Print and shaded views of the part. All mm, measured from the part's lowest x, y and z. A direction names the side the tool comes from. Round coordinates to 2 decimals unless told otherwise and drop trailing zeros. Order: outer loops, then holes, each group sorted by start corner. A loop starts at its lowest first (then second) coordinate and runs counter-clockwise, first axis right, second up. Notation, with made-up numbers: (77.25, 78.5) - (119.25, 78.5) arc R7 cw to (119.25, 82.5) - close; hole circle Ø5 at (51.25, 75). An arc over 180 degrees is marked (long way). Return JSON: item names as keys, results as strings. Group by question number.
Item 1: Saw through at C-C on z = 5. List the corners of the cut face in (x, y).
Item 2: Tool access for the marked faces 1, 2, 3, 4 and 5: list every direction of +Z, -Z, +X, -X, +Y, -Y with a clear straight run to the whole face (end or side of a thin tool).
Item 3: Saw through at A-A on x = 41. State how many separate pieces and enclosed holes the cut face has, and give its area (3 significant figures).
Item 4: Drop flat-ended pins along their axis: pin 1 (4 mm diameter, centred on x = 26.5, y = 19, fed in from +Z); pin 2 (3 mm diameter, centred on x = 8.5, y = 4, fed in from -Z); pin 3 (8 mm diameter, centred on x = 6.5, z = 33.5, fed in from -Y). Give the stop position or say it passes through.
Item 5: Saw through at B-B on y = 9. List the corners of the cut face in (x, z).
Item 6: Saw through at D-D on z = 30. List the corners of the cut face in (x, y).
Item 7: Probe probe 1 along Z at (x, y) = (21, 13.25); probe 2 along Y at (x, z) = (26.5, 19.5). List the from-to ranges inside material, lowest first.
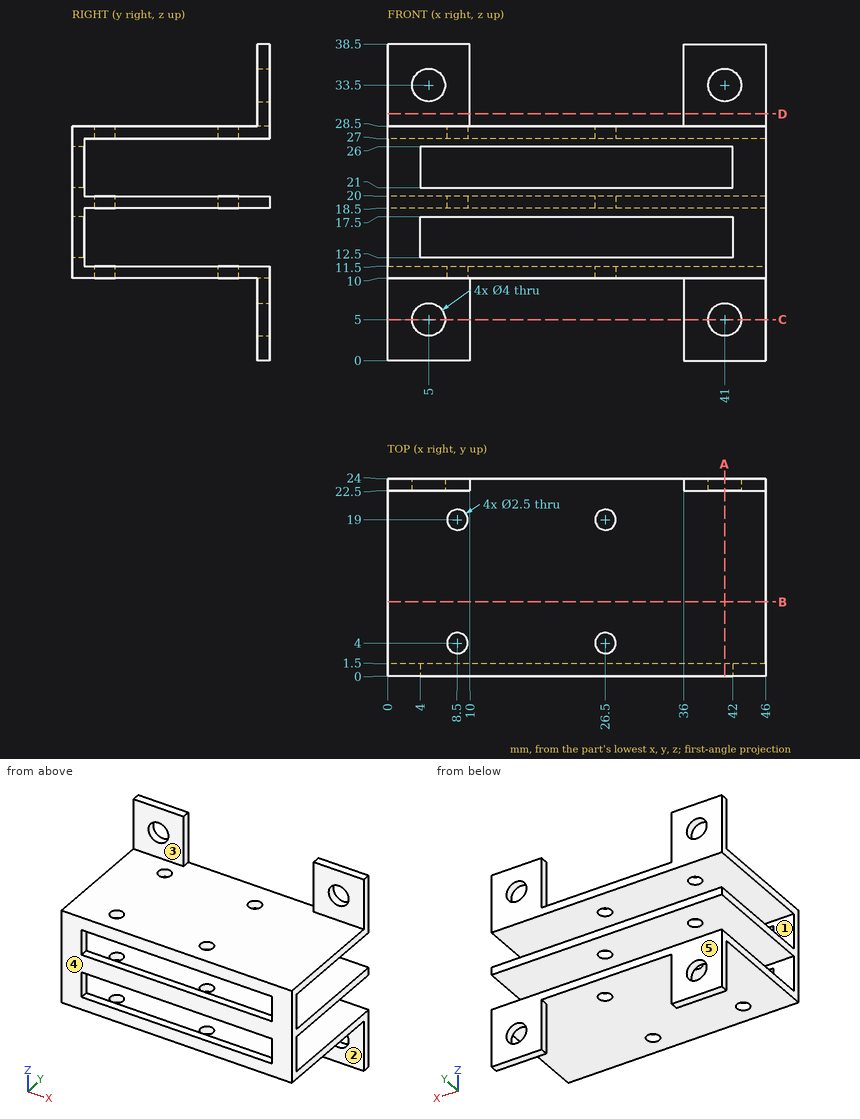
Filled in:
{
 "1": {"outline": "(0, 22.5) - (3, 22.5) - (3, 24) - (0, 24) - close; (7, 22.5) - (10, 22.5) - (10, 24) - (7, 24) - close; (36, 22.5) - (39, 22.5) - (39, 24) - (36, 24) - close; (43, 22.5) - (46, 22.5) - (46, 24) - (43, 24) - close"},
 "2": {"face 1": "+X, -X, +Y", "face 2": "-Z, +X, -X, -Y", "face 3": "+Z, +X, -X, -Y", "face 4": "+Z, -Z, +X, -X, -Y", "face 5": "+Z, -Z, +X, -X, +Y"},
 "3": {"separate pieces": "5", "enclosed holes": "0", "area": "132 mm^2"},
 "4": {"pin 1": "stops at z = 28.5", "pin 2": "stops at z = 10", "pin 3": "stops at y = 22.5"},
 "5": {"outline": "(0, 10) - (46, 10) - (46, 11.5) - (0, 11.5) - close; (0, 18.5) - (46, 18.5) - (46, 20) - (0, 20) - close; (0, 27) - (46, 27) - (46, 28.5) - (0, 28.5) - close"},
 "6": {"outline": "(0, 22.5) - (10, 22.5) - (10, 24) - (0, 24) - close; (36, 22.5) - (46, 22.5) - (46, 24) - (36, 24) - close"},
 "7": {"probe 1": "z = 10 to 11.5, 18.5 to 20, 27 to 28.5", "probe 2": "y = 0 to 2.75, 5.25 to 17.75, 20.25 to 24"}
}
